```python
from build123d import *

# Parameters (mm, degrees)
F0_R          = 6.223
F1_DEPTH      = 12.7
F3_R          = 7.62
F2_R          = 2.413
F4_DEPTH      = 17.781
F6_DEPTH      = 17.781
F8_DEPTH      = 6.35
F8_DEPTH_BACK = 5.081


with BuildPart() as f1:
    # F0 (on Front) → F1 (new body, symmetric)
    with BuildSketch(Plane.XZ):
        with BuildLine():
            Line((-6.35, 52.7261902376), (-6.35, 0))
            Line((-6.35, 0), (6.35, 0))
            Line((6.35, 0), (6.35, 52.7261902376))
            ThreePointArc((6.35, 52.7261902376), (0, 73.66), (-6.35, 52.7261902376))
        make_face()
        with Locations((0, 62.23)):
            Circle(F0_R, mode=Mode.SUBTRACT)
    extrude(amount=F1_DEPTH, both=True)

    # F3
    f3_edges = [f1.edges().sort_by_distance(p)[0] for p in [
        (-6.35, 0, 52.72619),
        (6.35, 0, 52.72619),
    ]]
    fillet(f3_edges, radius=F3_R)

    # F2 (on face) → F4 (cut, through all)
    with BuildSketch(Plane.YZ.offset(6.35)):
        with Locations((0, 36.83)):
            Circle(F2_R)
        with Locations((0, 13.97)):
            Circle(F2_R)
    extrude(amount=-F4_DEPTH, mode=Mode.SUBTRACT)

    # F5 (on face) → F6 (cut, through all)
    with BuildSketch(Plane.YZ.offset(6.35)):
        with BuildLine():
            ThreePointArc((2.413, 42.545), (0, 44.958), (-2.413, 42.545))
            Line((-2.413, 42.545), (-2.413, 31.115))
            ThreePointArc((-2.413, 31.115), (0, 28.702), (2.413, 31.115))
            Line((2.413, 31.115), (2.413, 42.545))
        make_face()
        with BuildLine():
            ThreePointArc((2.413, 19.685), (0, 22.098), (-2.413, 19.685))
            Line((-2.413, 19.685), (-2.413, 8.255))
            ThreePointArc((-2.413, 8.255), (0, 5.842), (2.413, 8.255))
            Line((2.413, 8.255), (2.413, 19.685))
        make_face()
    extrude(amount=-F6_DEPTH, mode=Mode.SUBTRACT)

    # F7 (on face) → F8 (cut, two sides)
    with BuildSketch(Plane.YZ.offset(6.35)) as f8_sk:
        with BuildLine():
            Line((4.572, 31.115), (4.572, 42.545))
            ThreePointArc((4.572, 42.545), (0, 47.117), (-4.572, 42.545))
            Line((-4.572, 42.545), (-4.572, 31.115))
            ThreePointArc((-4.572, 31.115), (0, 26.543), (4.572, 31.115))
        make_face()
        with BuildLine():
            Line((4.572, 8.255), (4.572, 19.685))
            ThreePointArc((4.572, 19.685), (0, 24.257), (-4.572, 19.685))
            Line((-4.572, 19.685), (-4.572, 8.255))
            ThreePointArc((-4.572, 8.255), (0, 3.683), (4.572, 8.255))
        make_face()
    extrude(amount=-F8_DEPTH, mode=Mode.SUBTRACT)
    extrude(f8_sk.sketch, amount=F8_DEPTH_BACK, mode=Mode.SUBTRACT)


solid = f1.part
```
Verification items for the finished model (mm, model axes). A direction names the side the tool comes from. Give positions to 0.01 mm unless a question says otherwise; leave off trailing zeros. Order: outer loops, then holes, each group sorted by start corner. A loop starts at its lowest first (then second) coordinate and runs counter-clockwise, first axis right, second up. Notation, with made-up numbers: M 66,86 L 101,86 A16 ccw 101,110 Z; hole C -29,25 d9. An arc over 180 degrees is marked long. Return JSON: item names as keys, results as strings. Group by question number.
1) Section check A-A on y = 0. Record the cut outline in (x, z), and give its area (3 significant figures).
2) Go/stop test with flat-tipped pins: pin 1 Ø5 at (x, y) = (-8, -8.5) entering from +Z; pin 2 Ø7.5 at (y, z) = (5.5, 15) entering from +X; pin 3 Ø2 at (x, y) = (-3.5, -9.5) entering from -Z; pin 4 Ø2.5 at (y, z) = (0.5, 34) entering from +X. Record where each tip stops, or that it passes through.
3) Section check C-C on x = -1.25. Record the cut outline in (y, z) (3 decimals).
4) Section check D-D on y = 5.5. Record the cut outline in (x, z), and give its area (3 significant figures).
5) Scan lines: line 1 (Z direction, x = 0, y = 5.5); line 2 (Z direction, x = -5.75, y = -0.5); line 3 (Y direction, x = 1.25, z = 10). Record each from-to range of solid material in increasing order.
6) Mould release check, pull along Z, two halves, no side actions. Record for faces 6 (the face through (0, -12.7, 37)), 7 (the face through (0, 0, 0)), 8 (the face through (-3.131, -0.053, 28.703)): pulls with the +Z half, pulls with the -Z half, needs draft (parallel to the pull), parting line crosses it, or undercut.
7) Section check B-B on z = 62.23. Record the cut outline in (x, y), and give its area (3 significant figures).
8) Access from +Z, -Z, +X, -X, +Y, -Y to the whole of each face (thin tool, end or side, straight path). Record for faces 1 (the face through (3.219, -0.101, 26.544)), 2 (the face through (-6.86, 0.18, 52.02)), 3 (the face through (-0.8, 0.2, 68.4)), 4 (the face through (6.35, -3, 24)), 5 (the face through (-3, 2.413, 37)).
Answer block:
{
 "1": {"outline": "M -8.38,54.46 A7.62 cw -6.35,49.28 L -6.35,44.96 L 0,44.96 L 0,47.12 L 6.35,47.12 L 6.35,49.28 A7.62 cw 8.38,54.46 A11.43 ccw long Z; M -6.35,0 L 6.35,0 L 6.35,3.68 L 0,3.68 L 0,5.84 L -6.35,5.84 Z; M -6.35,22.1 L 0,22.1 L 0,24.26 L 6.35,24.26 L 6.35,26.54 L 0,26.54 L 0,28.7 L -6.35,28.7 Z; hole C 0,62.23 d12.45", "area": "477 mm^2"},
 "2": {"pin 1": "stops at z = 72.25", "pin 2": "stops at x = 6.35", "pin 3": "stops at z = 0", "pin 4": "passes through"},
 "3": {"outline": "M -12.7,0 L 12.7,0 L 12.7,56.134 L -12.7,56.134 Z; M -12.7,68.326 L 12.7,68.326 L 12.7,73.591 L -12.7,73.591 Z; hole M -2.413,8.255 A2.413 ccw 2.413,8.255 L 2.413,19.685 A2.413 ccw -2.413,19.685 Z; hole M -2.413,31.115 A2.413 ccw 2.413,31.115 L 2.413,42.545 A2.413 ccw -2.413,42.545 Z"},
 "4": {"outline": "M -8.38,54.46 A7.62 cw -6.35,49.28 L -6.35,0 L 6.35,0 L 6.35,49.28 A7.62 cw 8.38,54.46 A11.43 ccw long Z; hole C 0,62.23 d12.45", "area": "945 mm^2"},
 "5": {"line 1": "z = 0 to 56.01, 68.45 to 73.66", "line 2": "z = 0 to 5.89, 22.05 to 28.75, 44.91 to 59.85, 64.61 to 72.11", "line 3": "y = -12.7 to -4.57, 4.57 to 12.7"},
 "6": {"face 6": "needs draft", "face 7": "pulls with the -Z half", "face 8": "undercut"},
 "7": {"outline": "M -11.43,-12.7 L -6.22,-12.7 L -6.22,12.7 L -11.43,12.7 Z; M 6.22,-12.7 L 11.43,-12.7 L 11.43,12.7 L 6.22,12.7 Z", "area": "265 mm^2"},
 "8": {"face 1": "+X", "face 2": "-Z, -X, +Y, -Y", "face 3": "+Y, -Y", "face 4": "-Z, +X, +Y, -Y", "face 5": "+X, -X"}
}
